from build123d import *

# Parameters (mm, degrees)
F0_W     = 3.175
F0_H     = 76.2
F0_W_2   = 69.85
F1_DEPTH = 1066.8
F5_W     = 69.85
F5_H     = 69.85
F6_DEPTH = 1066.801
F7_W     = 76.2
F7_H     = 76.6029041231
F8_DEPTH = 584.2


with BuildPart() as f1:
    # F0 (on Top) → F1 (new body)
    with BuildSketch(Plane.XY):
        with Locations((-36.5125, 0)):
            Rectangle(F0_W, F0_H)
        Rectangle(F0_W_2, F0_H)
        with Locations((36.5125, 0)):
            Rectangle(F0_W, F0_H)
    extrude(amount=F1_DEPTH)

    # F4: sweep along a path in F3
    with BuildLine(Plane.XZ) as f4_path:
        Line((38.2661430364, 38.2113192024), (468.4230136724, 0.577469484))
    # F2 (on face) → F4 (sweep)
    with BuildSketch(Plane.YZ.offset(38.1)):
        Polygon((-38.1, 0), (0, 0), (38.1, 0), (38.1, 76.2), (-38.1, 76.2), align=None)
        Polygon((31.75, 6.35), (0, 6.35), (-31.75, 6.35), (-31.75, 69.85), (31.75, 69.85), align=None, mode=Mode.SUBTRACT)
    sweep(path=f4_path.line)

    # F5 (on Top) → F6 (cut, through all)
    with BuildSketch(Plane.XY):
        Rectangle(F5_W, F5_H)
    extrude(amount=F6_DEPTH, mode=Mode.SUBTRACT)

    # F7 (on Top) → F8 (join)
    with BuildSketch(Plane.XY):
        with Locations((429.5848959012, -0.2014520615)):
            Rectangle(F7_W, F7_H)
    extrude(amount=-F8_DEPTH)


solid = f1.part
The listing builds one solid part. Answer for the finished solid, in the listing's coordinates (mm). A direction names the side the tool comes from. Give positions to 0.01 mm unless a question says otherwise; leave off trailing zeros. Loops run counter-clockwise (first coordinate to the right, second up) from the corner with the lowest first, then second, coordinate; pieces in that order, holes last.
Item 1: A cutting plane is placed at A-A (z = 404). Give the vertices of the cut face in (x, y) (3 decimals), then the cut area to 3 significant figures.
Derived:
outline: (-38.1, -38.1) - (38.1, -38.1) - (38.1, 38.1) - (-38.1, 38.1) - close; hole (-34.925, -34.925) - (34.925, -34.925) - (34.925, 34.925) - (-34.925, 34.925) - close
area: 927 mm2
Item 2: A cutting plane is placed at D-D (z = -70). Give the vertices of the cut face in (x, y), then the cut area to 3 significant figures.
Derived:
outline: (391.48, -38.5) - (467.68, -38.5) - (467.68, 38.1) - (391.48, 38.1) - close
area: 5,840 mm2
Item 3: A tool of negligible diameter and unlimited length cuts with its end or side. For faces 1 (the flat face through (429, 0, -584.2)), 2 (the flat face through (256, 31.75, 20)), 3 (the flat face through (38.1, -1, 565)), 4 (the flat face through (0, 34.925, 526)), from which of +Z, -Z, +X, -X, +Y, -Y can it reach the whole face along a straight path? Write none if from no direction.
Derived:
face 1: -Z, +X, -X, +Y, -Y
face 2: none
face 3: +Z, +X, +Y, -Y
face 4: +Z, -Z
Item 4: Find the intervals of material crossed by line 1 along X through (y, z) = (-14, 844) (3 decimals); line 2 along X through (y, z) = (-11, -499), in increasing order.
Derived:
line 1: x = -38.1 to -34.925, 34.925 to 38.1
line 2: x = 391.48 to 467.68
Item 5: A cutting plane is placed at C-C (x = 179.5). Give the vertices of the cut face in (y, z).
Derived:
outline: (-38.1, -12.37) - (38.1, -12.37) - (38.1, 63.83) - (-38.1, 63.83) - close; hole (-31.75, -6.02) - (31.75, -6.02) - (31.75, 57.48) - (-31.75, 57.48) - close
Item 6: A cutting plane is placed at B-B (y = 6). Give the vertices of the cut face in (x, z) (3 decimals), then the cut area to 3 significant figures.
Derived:
outline: (-38.1, 0) - (-34.925, 0) - (-34.925, 1066.8) - (-38.1, 1066.8) - close; (34.925, 0) - (38.1, 0) - (391.485, -30.917) - (391.485, -584.2) - (467.685, -584.2) - (467.685, -37.584) - (468.257, -37.634) - (468.257, -31.284) - (467.685, -31.234) - (467.685, 0) - (391.485, 0) - (391.485, -24.567) - (38.1, 6.35) - (38.1, 69.85) - (468.257, 32.216) - (468.257, 38.566) - (38.1, 76.2) - (38.1, 1066.8) - (34.925, 1066.8) - close
area: 56,300 mm2
Item 7: Determine the mould class of faces 5 (the flat face through (38.1, 0, 38)), 6 (the flat face through (-3, -37, 1066.8)), 7 (the flat face through (429, -38.503, -288)) for opening direction Z: +Z half, -Z half, draft (parallel to the pull), parting line (faces both ways), or undercut.
Derived:
face 5: undercut
face 6: +Z half
face 7: draft
Item 8: Each of these flat-tipped pins is pushed along its axis until it touches: pin 1 Ø19 at (x, y) = (411, -15.5) entering from +Z; pin 2 Ø23 at (y, z) = (-17, 789.5) entering from +X; pin 3 Ø4 at (x, y) = (136.5, 27.5) entering from +Z. Where does it stop, or does it pass through?
Derived:
pin 1: stops at z = 44.41
pin 2: stops at x = 38.1
pin 3: stops at z = 67.77
